Check sheet for the modelled part. Datum: model origin and axes. Units: mm. A direction names the side the tool comes from. Coordinates: 2 decimals unless noted, no trailing zeros. Loops run counter-clockwise (first coordinate to the right, second up) from the corner with the lowest first, then second, coordinate; pieces in that order, holes last. Notation, with made-up numbers: (31.5, -21) - (65.5, -21) arc R35 cw to (65.5, 14) - close; hole circle Ø1 at (9, 35). An arc over 180 degrees is marked (long way). Write each question's results on one line, items separated by ' | '. Start each with the question number.
1. Cross-section at A-A (z = 28). Record the cut outline in (x, y).
2. Cross-section at D-D (x = -7.62). Record the cut outline in (y, z) (3 decimals).
3. Cross-section at B-B (y = -12). Record the cut outline in (x, z).
4. Gauge pin test, flat ends, axial feed: P1, Ø3, axis at x = -25.4, y = 0, coming from the -Z side; P2, Ø3, axis at x = -34, z = -23.5, coming from the -Y side. Record the tip position at first contact, or that the pin passes through.
5. Tool access check on faces 1 (the face through (-72.633, 0.533, -34.281)), 2 (the face through (-10.65, -0.95, -44.54)), 3 (the face through (-1, 63.476, 4)). Record the directions out of +Z, -Z, +X, -X, +Y, -Y that give a thin tool (end or side, any length) a straight path to the whole face; none if there is none.
6. Draft check along X on faces 4 (the face through (-1, 1, -50.8)), 5 (the face through (-88.935, 1, 6)), 6 (the face through (-72.435, 47.119, 12.167)). Enter one of: released by +X, released by -X, zero draft, split by the parting line, or undercut.
7. Thickness scan on line 1 (Z direction, x = -29, y = -38.5); line 2 (Y direction, x = -25.4, z = -42.75); line 3 (X direction, y = 12, z = 7). Record the ranges inside material, lowest first. Write a range as [from, to].
8. Cross-section at C-C (x = -42). Record the cut outline in (y, z), and give its area (3 significant figures).
```python
from build123d import *

# Parameters (mm, degrees)
BOSS_EXTRUDE1_DEPTH      = 50.8
BOSS_EXTRUDE1_DEPTH_BACK = 50.8
SKETCH1_W                = 177.870967952
SKETCH1_H                = 126.951722988
SKETCH3_W                = 152.508374468
SKETCH3_H                = 101.481852174
CUT_EXTRUDE1_DEPTH       = 88.9
FILLET1_R                = 12.7
CUT_EXTRUDE2_DEPTH       = 138.938
CUT_EXTRUDE2_DEPTH_BACK  = 127
SKETCH4_R                = 1.5875
CUT_EXTRUDE3_DEPTH       = 141.861333596
CUT_EXTRUDE3_DEPTH_BACK  = 36.576
SKETCH5_R                = 3.175
SKETCH6_W                = 177.870967952
SKETCH6_H                = 10.163315621
BOSS_EXTRUDE2_DEPTH      = 127


with BuildPart() as part:
    # Sketch1 → Boss-Extrude1 (new, two sides: drawn at the far end of the back side and taken through both)
    with BuildSketch(Plane.XY.offset(-BOSS_EXTRUDE1_DEPTH_BACK)):
        Rectangle(SKETCH1_W, SKETCH1_H)
    extrude(amount=BOSS_EXTRUDE1_DEPTH + BOSS_EXTRUDE1_DEPTH_BACK)

    # Sketch3 → Cut-Extrude1 (cut)
    with BuildSketch(Plane.XY.offset(50.8)):
        Rectangle(SKETCH3_W, SKETCH3_H)
    extrude(amount=-CUT_EXTRUDE1_DEPTH, mode=Mode.SUBTRACT)

    # Fillet1
    fillet1_edges = [part.edges().sort_by_distance(p)[0] for p in [
        (76.254187234, 0, -38.1),
        (76.254187234, 50.740926087, 6.35),
        (0, -50.740926087, -38.1),
        (76.254187234, -50.740926087, 6.35),
        (-76.254187234, 0, -38.1),
        (-76.254187234, -50.740926087, 6.35),
        (0, 50.740926087, -38.1),
        (-76.254187234, 50.740926087, 6.35),
    ]]
    fillet(fillet1_edges, radius=FILLET1_R)

    # Sketch4 → Cut-Extrude2 (cut, two sides: drawn at the far end of the back side and taken through both)
    with BuildSketch(Plane.XY.offset(-38.1).offset(-CUT_EXTRUDE2_DEPTH_BACK)):
        with Locations(Location((-25.4, 0, 0), (0, 0, 180))):
            Circle(SKETCH4_R)
    extrude(amount=CUT_EXTRUDE2_DEPTH + CUT_EXTRUDE2_DEPTH_BACK, mode=Mode.SUBTRACT)

    # Sketch5 → Cut-Extrude3 (cut, two sides: drawn at the far end of the back side and taken through both)
    with BuildSketch(Plane.XY.offset(-38.1).offset(-CUT_EXTRUDE3_DEPTH_BACK)):
        with Locations(Location((-7.62, 0, 0), (0, 0, 180))):
            Circle(SKETCH5_R)
    extrude(amount=CUT_EXTRUDE3_DEPTH + CUT_EXTRUDE3_DEPTH_BACK, mode=Mode.SUBTRACT)

    # Sketch6 → Boss-Extrude2 (add)
    with BuildSketch(Plane(origin=(0, 63.475861494, 0), x_dir=(1, 0, 0), z_dir=(0, 1, 0))):
        with Locations((0, -55.881657811)):
            Rectangle(SKETCH6_W, SKETCH6_H)
    extrude(amount=-BOSS_EXTRUDE2_DEPTH)


solid = part.part
```
Established:
1) outline: (-88.94, -63.48) - (88.94, -63.48) - (88.94, 63.48) - (-88.94, 63.48) - close; hole (-76.25, -38.04) arc R12.7 ccw to (-63.55, -50.74) - (63.55, -50.74) arc R12.7 ccw to (76.25, -38.04) - (76.25, 38.04) arc R12.7 ccw to (63.55, 50.74) - (-63.55, 50.74) arc R12.7 ccw to (-76.25, 38.04) - close
2) outline: (-63.524, 50.8) - (-63.476, 50.8) - (-63.476, -50.8) - (-3.175, -50.8) - (-3.175, -38.1) - (-38.041, -38.1) arc R12.7 cw to (-50.741, -25.4) - (-50.741, 50.8) - (50.741, 50.8) - (50.741, -25.4) arc R12.7 cw to (38.041, -38.1) - (3.175, -38.1) - (3.175, -50.8) - (63.476, -50.8) - (63.476, 60.963) - (-63.524, 60.963) - close
3) outline: (-88.94, -50.8) - (88.94, -50.8) - (88.94, 60.96) - (-88.94, 60.96) - close; hole (-76.25, -25.4) arc R12.7 ccw to (-63.55, -38.1) - (63.55, -38.1) arc R12.7 ccw to (76.25, -25.4) - (76.25, 50.8) - (-76.25, 50.8) - close
4) P1: z = 50.8 | P2: y = -63.48
5) face 1: none | face 2: -Z | face 3: +Z, -Z, +X, -X, +Y
6) face 4: zero draft | face 5: released by -X | face 6: undercut
7) line 1: [-50.8, -38.09], [50.8, 60.96] | line 2: [-63.48, -1.59], [1.59, 63.48] | line 3: [-88.94, -76.25], [76.25, 88.94]
8) outline: (-63.52, 50.8) - (-63.48, 50.8) - (-63.48, -50.8) - (63.48, -50.8) - (63.48, 60.96) - (-63.52, 60.96) - close; hole (-50.74, -25.4) arc R12.7 ccw to (-38.04, -38.1) - (38.04, -38.1) arc R12.7 ccw to (50.74, -25.4) - (50.74, 50.8) - (-50.74, 50.8) - close | area: 5,240 mm^2
